Autodesk Inventor part; units mm, degrees
ref_plane "Work Plane1" through (-19.25, -0.5, 9.85) normal (0, 0, 1) x (1, 0, 0)
ref_plane "Work Plane2" through (-19.25, -0.5, 12.85) normal (0, 0, 1) x (1, 0, 0)
ref_plane "Work Plane4" through (19.95, -28.3, 9.85) normal (1, 0, 0) x (0, 0, -1)
ref_plane "Work Plane1" through (-19.25, -0.5, 9.85) normal (0, 0, 1) x (1, 0, 0)
sketch "Sketch1" plane through (-19.25, -0.5, 9.85) normal (0, 0, 1) x (1, 0, 0)
  line L0 (-0.695, -27.8) -> (39.2, -27.8)
  line L1 (39.2, -27.8) -> (39.2, 8.9608)
  line L2 (39.2, 8.9608) -> (-0.695, 8.9608)
  line L3 (-0.695, 8.9608) -> (-0.695, -27.8)
  point P0 (19.25, 0.5)
extrude "Extrusion1" add sketch "Sketch1" along normal blind 3
ref_plane "Work Plane2" through (-19.25, -0.5, 12.85) normal (0, 0, 1) x (1, 0, 0)
sketch "Sketch2" plane through (-19.25, -0.5, 12.85) normal (0, 0, 1) x (1, 0, 0)
  line L0 (39.2, -27.8) -> (39.2, 8.9608)
  line L1 (39.2, -27.8) -> (-0.695, -27.8)
  line L2 (-0.695, -27.8) -> (-0.695, 8.9608)
  line L3 (-0.695, 8.9608) -> (39.2, 8.9608)
  line L4 (39.2, 8.9608) -> (39.2, -27.8)
  point P0 (19.25, 0.5)
  point P1 (39.2, 8.9608)
extrude "Extrusion2" add sketch "Sketch2" along normal blind 5
ref_plane "Work Plane4" through (19.95, -28.3, 9.85) normal (1, 0, 0) x (0, 0, -1)
sketch "Sketch3" plane through (19.95, -28.3, 9.85) normal (1, 0, 0) x (0, 0, -1)
  line L0 (0, 0) -> (0, 36.7608)
  line L1 (0, 0) -> (-8, 0)
  line L2 (0, 36.7608) -> (-2, 36.7608)
  line L3 (-2, 36.7608) -> (-2, 0)
  line L4 (-2, 0) -> (0, 0)
  line L5 (0, 0) -> (0, 36.7608)
  point P0 (9.85, 28.3)
  dimension "d4" = 2
extrude "Extrusion3" cut sketch "Sketch3" against normal blind 50
ref_plane "Work Plane3" through (19.95, -28.3, 17.85) normal (1, 0, 0) x (0, 0, -1)
sketch "Sketch4" plane through (19.95, -28.3, 17.85) normal (1, 0, 0) x (0, 0, -1)
  line L0 (6, 0) -> (0, 0)
  line L1 (6, 36.7608) -> (0, 36.7608)
  line L2 (0, 0) -> (1, 0)
  line L3 (1, 0) -> (1, 36.7608)
  line L4 (1, 36.7608) -> (0, 36.7608)
  line L5 (0, 36.7608) -> (0, 0)
  point P0 (17.85, 28.3)
  point P1 (1, 0)
  dimension "d7" = 1
extrude "Extrusion4" cut sketch "Sketch4" against normal blind 50
ref_plane "Work Plane5" through (19.95, -28.3, 11.85) normal (1, 0, 0) x (0, 0, -1)
sketch "Sketch5" plane through (19.95, -28.3, 11.85) normal (1, 0, 0) x (0, 0, -1)
  line L0 (-5, 36.7608) -> (-5, 0)
  line L1 (0, 0) -> (0, 36.7608)
  line L2 (-5, 36.7608) -> (0, 36.7608)
  line L3 (0, 36.7608) -> (0, 0)
  line L4 (0, 0) -> (-5, 0)
  line L5 (-5, 0) -> (-5, 36.7608)
  point P0 (11.85, 28.3)
extrude "Extrusion5" add sketch "Sketch5" along normal blind 7
ref_plane "Work Plane6" through (-19.945, -28.3, 11.85) normal (0, 0, -1) x (-1, 0, 0)
sketch "Sketch6" plane through (-19.945, -28.3, 11.85) normal (0, 0, -1) x (-1, 0, 0)
  line L0 (-46.895, 0) -> (-46.895, 36.7608)
  line L1 (-46.895, 27.8459) -> (-40.895, 27.8459)
  line L2 (-40.895, 27.8459) -> (-40.895, 11.8459)
  line L3 (-40.895, 11.8459) -> (-46.895, 11.8459)
  line L4 (-46.895, 11.8459) -> (-46.895, 27.8459)
  point P0 (-19.945, 28.3)
  dimension "d12" = 6
  dimension "d13" = 16
extrude "Extrusion6" add sketch "Sketch6" along normal blind 22.875
sketch "Sketch7" plane through (20.95, -0.4541, 11.85) normal (0, 1, 0) x (1, 0, 0)
  arc A0 (5.4164, 8.2173) -> (5.4164, 5.6327) centre (3.7611, 6.925) ccw
  circle A1 centre (3.7611, 6.925) radius 2.5
  arc A2 (5.4164, 18.0673) -> (5.4164, 15.4827) centre (3.7611, 16.775) ccw
  circle A3 centre (3.7611, 16.775) radius 2.5
  point P0 (-20.95, 11.85)
  dimension "d16" = 5
  dimension "d17" = 5
extrude "Extrusion7" cut sketch "Sketch7" against normal blind 22.875
ref_plane "Work Plane7" through (26.95, -28.3, 11.85) normal (1, 0, 0) x (0, 0, -1)
sketch "Sketch8" plane through (26.95, -28.3, 11.85) normal (1, 0, 0) x (0, 0, -1)
  line L0 (0, 11.8459) -> (22.875, 11.8459)
  line L1 (22.875, 27.8459) -> (22.875, 11.8459)
  line L2 (0, 11.8459) -> (22.875, 11.8459)
  line L3 (22.875, 11.8459) -> (22.875, 16.8459)
  line L4 (22.875, 16.8459) -> (0, 16.8459)
  line L5 (0, 16.8459) -> (0, 11.8459)
  point P0 (11.85, 28.3)
  dimension "d20" = 5
extrude "Extrusion8" cut sketch "Sketch8" against normal blind 6.7
ref_plane "Work Plane8" through (-19.945, -28.3, 11.85) normal (-1, 0, 0) x (0, 0, 1)
sketch "Sketch9" plane through (-19.945, -28.3, 11.85) normal (-1, 0, 0) x (0, 0, 1)
  line L0 (0, 36.7608) -> (0, 0)
  line L1 (5, 0) -> (0, 0)
  line L2 (0, 36.7608) -> (5, 36.7608)
  line L3 (5, 36.7608) -> (5, 0)
  line L4 (5, 0) -> (0, 0)
  line L5 (0, 0) -> (0, 36.7608)
  point P0 (-11.85, 28.3)
extrude "Extrusion9" add sketch "Sketch9" along normal blind 7
ref_plane "Work Plane10" through (26.95, -0.4541, 11.85) normal (0, 0, -1) x (-1, 0, 0)
sketch "Sketch11" plane through (26.95, -0.4541, 11.85) normal (0, 0, -1) x (-1, 0, 0)
  line L0 (53.895, -27.8459) -> (53.895, 8.9148)
  line L1 (53.895, 0) -> (47.895, 0)
  line L2 (47.895, 0) -> (47.895, -11)
  line L3 (47.895, -11) -> (53.895, -11)
  line L4 (53.895, -11) -> (53.895, 0)
  point P0 (26.95, 0.4541)
  dimension "d25" = 6
extrude "Extrusion10" add sketch "Sketch11" along normal blind 22.875
sketch "Sketch12" plane through (-26.945, -0.4541, 11.85) normal (0, 1, 0) x (1, 0, 0)
  arc A0 (0.5786, 15.4827) -> (0.5786, 18.0673) centre (2.2339, 16.775) ccw
  circle A1 centre (2.2339, 16.775) radius 2.5
  arc A2 (0.5786, 5.6327) -> (0.5786, 8.2173) centre (2.2339, 6.925) ccw
  circle A3 centre (2.2339, 6.925) radius 2.5
  point P0 (26.945, 11.85)
  dimension "d28" = 5
  dimension "d29" = 5
extrude "Extrusion11" cut sketch "Sketch12" against normal blind 22.875
ref_plane "Work Plane11" through (-26.945, -28.3, 11.85) normal (-1, 0, 0) x (0, 0, 1)
sketch "Sketch13" plane through (-26.945, -28.3, 11.85) normal (-1, 0, 0) x (0, 0, 1)
  line L0 (0, 16.8459) -> (0, 27.8459)
  line L1 (5, 36.7608) -> (0, 36.7608)
  line L2 (0, 27.8459) -> (5, 27.8459)
  line L3 (5, 27.8459) -> (5, 36.7608)
  line L4 (5, 36.7608) -> (0, 36.7608)
  line L5 (0, 36.7608) -> (0, 27.8459)
  point P0 (-11.85, 28.3)
extrude "Extrusion12" cut sketch "Sketch13" against normal blind 67.325
ref_plane "Work Plane9" through (26.95, -28.3, 11.85) normal (0, -1, 0) x (1, 0, 0)
sketch "Sketch14" plane through (26.95, -28.3, 11.85) normal (0, -1, 0) x (1, 0, 0)
  line L0 (0, 5) -> (0, 0)
  line L1 (0, 5) -> (-53.895, 5)
  line L2 (0, 0) -> (-53.895, 0)
  line L3 (-53.895, 0) -> (-53.895, 5)
  line L4 (-53.895, 5) -> (0, 5)
  line L5 (0, 5) -> (0, 0)
  point P0 (-26.95, -11.85)
extrude "Extrusion13" add sketch "Sketch14" along normal blind 5
ref_plane "Work Plane12" through (26.95, -11.4541, 11.85) normal (0, 0, -1) x (-1, 0, 0)
sketch "Sketch15" plane through (26.95, -11.4541, 11.85) normal (0, 0, -1) x (-1, 0, 0)
  line L0 (53.895, -21.8459) -> (0, -21.8459)
  line L1 (53.895, 11) -> (53.895, -21.8459)
  line L2 (0, -21.8459) -> (53.895, -21.8459)
  line L3 (53.895, -21.8459) -> (53.895, -17.8459)
  line L4 (53.895, -17.8459) -> (0, -17.8459)
  line L5 (0, -17.8459) -> (0, -21.8459)
  point P0 (26.95, 11.4541)
  dimension "d36" = 4
extrude "Extrusion14" add sketch "Sketch15" along normal blind 22.4625
ref_plane "Work Plane13" through (-26.945, -29.3, 11.85) normal (0, 1, 0) x (1, 0, 0)
sketch "Sketch16" plane through (-26.945, -29.3, 11.85) normal (0, 1, 0) x (1, 0, 0)
  line L0 (53.895, 0) -> (53.895, 22.4625)
  line L1 (0, 0) -> (0, 22.4625)
  line L2 (53.895, 0) -> (0, 0)
  line L3 (0, 0) -> (0, 1)
  line L4 (0, 1) -> (53.895, 1)
  line L5 (53.895, 1) -> (53.895, 0)
  point P0 (26.945, 11.85)
  point P1 (53.895, 1)
  dimension "d39" = 1
extrude "Extrusion15" add sketch "Sketch16" along normal blind 30
ref_plane "Work Plane14" through (26.95, -28.3, 11.85) normal (1, 0, 0) x (0, 0, -1)
sketch "Sketch17" plane through (26.95, -28.3, 11.85) normal (1, 0, 0) x (0, 0, -1)
  line L0 (0, 29) -> (1, 29)
  line L1 (5.8126, 27.8459) -> (1, 27.8459)
  line L2 (0, 29) -> (1, 29)
  line L3 (1, 29) -> (1, 27.8459)
  line L4 (1, 27.8459) -> (0, 27.8459)
  line L5 (0, 27.8459) -> (0, 29)
  point P0 (11.85, 28.3)
extrude "Extrusion16" cut sketch "Sketch17" against normal blind 100
sketch "Sketch19" plane through (26.95, -33.3, 11.85) normal (0, -1, 0) x (1, 0, 0)
  circle A0 centre (-16.85, -11.85) radius 5
  circle A1 centre (-16.85, -11.85) radius 1.5
  point P0 (-26.95, -11.85)
  dimension "d47" = 10
  dimension "d50" = 3
extrude "Extrusion20" cut sketch "Sketch19" against normal blind 10 contours A1
sketch "Sketch20" plane through (26.95, -33.3, 11.85) normal (0, -1, 0) x (1, 0, 0)
  line L0 (-53.895, -22.4625) -> (0, -22.4625)
  line L1 (-53.895, 5) -> (-53.895, -22.4625)
  line L2 (0, -22.4625) -> (-53.895, -22.4625)
  line L3 (-53.895, -22.4625) -> (-53.895, 5)
  line L4 (-53.895, 5) -> (0, 5)
  line L5 (0, 5) -> (0, -22.4625)
  point P0 (-26.95, -11.85)
extrude "Extrusion21" add sketch "Sketch20" along normal blind 2
sketch "Sketch21" plane through (-26.945, -29.3, -10.6125) normal (0, 1, 0) x (1, 0, 0)
  circle A0 centre (37.045, -10.6125) radius 1.5
  circle A1 centre (37.045, -10.6125) radius 1.5
  point P0 (26.945, -10.6125)
extrude "Extrusion22" cut sketch "Sketch21" against normal blind 10
sketch "Sketch22" plane through (-26.945, -29.3, -10.6125) normal (0, 1, 0) x (1, 0, 0)
  circle A0 centre (37.045, -10.6125) radius 1.5
  circle A1 centre (37.045, -10.6125) radius 2.5
  point P0 (26.945, -10.6125)
  dimension "d59" = 5
extrude "Extrusion23" cut sketch "Sketch22" against normal blind 2
sketch "Sketch23" plane through (-19.945, -28.3, -11.025) normal (0, 0, -1) x (-1, 0, 0)
  line L0 (-46.895, 27.8459) -> (-46.895, 16.8459)
  line L1 (-46.895, 27.8459) -> (-48.895, 27.8459)
  line L2 (-48.895, 27.8459) -> (-48.895, 16.8459)
  line L3 (-48.895, 16.8459) -> (-46.895, 16.8459)
  line L4 (-46.895, 16.8459) -> (-46.895, 27.8459)
  line L5 (7, 16.8459) -> (7, 27.8459)
  line L6 (7, 27.8459) -> (9, 27.8459)
  line L7 (9, 27.8459) -> (9, 16.8459)
  line L8 (9, 16.8459) -> (7, 16.8459)
  line L9 (7, 16.8459) -> (7, 27.8459)
  point P0 (-19.945, 28.3)
  dimension "d62" = 2
  dimension "d63" = 2
extrude "Extrusion24" add sketch "Sketch23" against normal up to surface (27.875 mm away)
sketch "Sketch24" plane through (-20.945, -0.4541, 10.85) normal (0, 1, 0) x (1, 0, 0)
  arc A0 (47.895, 7.0374) -> (47.895, 4.8126) centre (45.6561, 5.925) ccw
  circle A1 centre (45.6561, 5.925) radius 1.6
  arc A2 (47.895, 16.8874) -> (47.895, 14.6626) centre (45.6561, 15.775) ccw
  circle A3 centre (45.6561, 15.775) radius 1.6
  circle A4 centre (45.6561, 5.925) radius 2.5
  circle A5 centre (45.6561, 15.775) radius 2.5
  point P0 (20.945, 10.85)
  point P1 (47.895, 4.8126)
  dimension "d66" = 3.2
  dimension "d67" = 3.2
extrude "Extrusion25" add sketch "Sketch24" against normal up to surface (11 mm away)
sketch "Sketch25" plane through (-20.945, -0.4541, 10.85) normal (0, 1, 0) x (1, 0, 0)
  arc A0 (-6, 4.8025) -> (-6, 7.0475) centre (-3.7661, 5.925) ccw
  circle A1 centre (-3.7661, 5.925) radius 1.6
  arc A2 (-6, 14.6525) -> (-6, 16.8975) centre (-3.7661, 15.775) ccw
  circle A3 centre (-3.7661, 15.775) radius 1.6
  circle A4 centre (-3.7661, 15.775) radius 2.5
  circle A5 centre (-3.7661, 5.925) radius 2.5
  point P0 (20.945, 10.85)
  point P1 (-6, 7.0475)
  dimension "d70" = 3.2
  dimension "d71" = 3.2
  dimension "d72" = 5
  dimension "d73" = 5
extrude "Extrusion26" add sketch "Sketch25" against normal up to surface (11 mm away)
sketch "Sketch26" plane through (26.95, -35.3, 11.85) normal (0, -1, 0) x (1, 0, 0)
  line L0 (-55.895, -22.875) -> (-55.895, 5)
  line L1 (-55.895, -11.85) -> (-37.045, -11.85)
  line L2 (-55.895, -11.85) -> (-37.045, -11.85) construction
  circle A0 centre (-37.045, -11.85) radius 1.5
  point P0 (-26.95, -11.85)
  dimension "d76" = 18.85
  dimension "d77" = 0
  dimension "d78" = 3
extrude "Extrusion27" cut sketch "Sketch26" against normal blind 10
sketch "Sketch27" plane through (-26.945, -29.3, -10.6125) normal (0, 1, 0) x (1, 0, 0)
  circle A0 centre (16.85, -10.6125) radius 1.5
  circle A1 centre (16.85, -10.6125) radius 2.5
  point P0 (26.945, -10.6125)
  dimension "d81" = 5
extrude "Extrusion28" cut sketch "Sketch27" against normal up to surface (2 mm away)
sketch "Sketch28" plane through (-26.945, -35.3, 16.85) normal (0, 0, 1) x (1, 0, 0)
  line L0 (0, 0) -> (53.895, 0)
  line L1 (26.9475, 0) -> (26.9475, 34.8459)
  line L2 (6, 34.8459) -> (47.895, 34.8459)
  point P0 (26.945, 35.3)
sketch "Sketch29" plane through (-26.945, -11.4541, 10.85) normal (0, -1, 0) x (1, 0, 0)
  line L0 (6, 0) -> (0, 0)
  line L1 (-2, 6) -> (0, 6)
  line L2 (0, 0) -> (-2, 0)
  line L3 (-2, 0) -> (-2, 6)
  line L4 (-2, 6) -> (0, 6)
  line L5 (0, 6) -> (0, 0)
  line L6 (53.895, 0) -> (53.895, 6)
  line L7 (55.895, -21.875) -> (55.895, 6)
  line L8 (53.895, 0) -> (55.895, 0)
  line L9 (55.895, 0) -> (55.895, 6)
  line L10 (55.895, 6) -> (53.895, 6)
  line L11 (53.895, 6) -> (53.895, 0)
  point P0 (26.945, -10.85)
extrude "Extrusion29" add sketch "Sketch29" along normal up to surface (23.8459 mm away)
sketch "Sketch30" plane through (26.95, -29.3, 10.85) normal (0, 0, -1) x (-1, 0, 0)
  line L0 (53.895, 0) -> (0, 0)
  line L1 (-2, -6) -> (0, -6)
  line L2 (0, 0) -> (-2, 0)
  line L3 (-2, 0) -> (-2, -6)
  line L4 (-2, -6) -> (0, -6)
  line L5 (0, -6) -> (0, 0)
  line L6 (55.895, -6) -> (-2, -6)
  line L7 (55.895, 17.8459) -> (55.895, -6)
  line L8 (53.895, -6) -> (55.895, -6)
  line L9 (55.895, -6) -> (55.895, 0)
  line L10 (55.895, 0) -> (53.895, 0)
  line L11 (53.895, 0) -> (53.895, -6)
  point P0 (26.95, 29.3)
extrude "Extrusion30" add sketch "Sketch30" along normal up to surface (21.4625 mm away) contours L10 L7 L6 L11 | L5 L1 L3 L2
properties part number "MG996RServoHolder" material "钢"
For this review, take the finished solid that the model builds, in its own axes (mm). A direction names the side the tool comes from. Give positions to 0.01 mm unless a question says otherwise; leave off trailing zeros. Loops run counter-clockwise (first coordinate to the right, second up) from the corner with the lowest first, then second, coordinate; pieces in that order, holes last. Notation, with made-up numbers: M 7.5,57.5 L 61.5,57.5 A26 ccw 61.5,78.5 Z; hole C 36,-29 d4. An arc over 180 degrees is marked long. Answer as a JSON object with one key per item and string values. Group by question number.
Q1. Mouldability with a two-part tool opening along Z and no side actions: class faces 1 (the cylindrical face through (23.532, -5.877, 3.844)), 2 (the flat face through (28.95, -10, 6)), 3 (the flat face through (0, -15, 10.85)) as +Z half, -Z half, draft (parallel to the pull), parting line (faces both ways), or undercut.
Q2. Add section B-B on x = 10.1. Give the boundary of the cut face in (y, z).
Q3. Add section C-C on y = -5.5. Give the boundary of the cut face in (x, z) (3 decimals).
Q4. Add section D-D on x = 20. Give the boundary of the cut face in (y, z), and give its area (3 significant figures).
Q5. Tool access review of faces 4 (the flat face through (0, -0.454, 12)), 5 (the flat face through (0, -29.3, 0)), 6 (the cylindrical face through (-23.973, -5.877, -3.506)), 7 (the flat face through (0, -32, -10.612)): name each direction out of +Z, -Z, +X, -X, +Y, -Y from which nothing blocks a thin tool from reaching the whole face with its end or side.
Q6. Insertion check: P1, Ø2.5, axis at x = -24.71, z = 4.92, coming from the +Y side; P2, Ø1.8, axis at x = 10.1, z = 0, coming from the +Y side; P3, Ø14.5, axis at x = 0, y = -8, coming from the -Z side; P4, Ø1.5, axis at x = -9.5, z = 1, coming from the +Y side. Each pin has a flat end and moves straight along its axis. Give the tip position at first contact, or say it passes through.
Q7. For probe 1 along X at (y, z) = (-34.2, 0) (3 decimals); probe 2 along Y at (x, z) = (26, 0.75); probe 3 along X at (y, z) = (-4, 2.75) (3 decimals), list the stretches that pass through material, from the lowest coordinate up. Write a range as [from, to].
Q8. Add section A-A on z = 0. Give the boundary of the cut face in (x, y) (3 decimals), and give its area (3 significant figures).
Checked values:
{
 "1": {"face 1": "undercut", "face 2": "draft", "face 3": "-Z half"},
 "2": {"outline": "M -35.3,-10.61 L -29.3,-10.61 L -29.3,-2.5 L -31.3,-2.5 L -31.3,-1.5 L -35.3,-1.5 Z; M -35.3,1.5 L -31.3,1.5 L -31.3,2.5 L -29.3,2.5 L -29.3,10.85 L -0.45,10.85 L -0.45,16.85 L -35.3,16.85 Z"},
 "3": {"outline": "M -28.945,-11.025 L -20.945,-11.025 L -20.945,10.85 L 20.95,10.85 L 20.95,-11.025 L 28.95,-11.025 L 28.95,16.85 L -28.945,16.85 Z; hole C -24.711,-4.925 d3.2; hole C -24.711,4.925 d3.2; hole C 24.711,-4.925 d3.2; hole C 24.711,4.925 d3.2"},
 "4": {"outline": "M -35.3,-10.61 L -29.3,-10.61 L -29.3,10.85 L -0.45,10.85 L -0.45,16.85 L -35.3,16.85 Z", "area": "338 mm²"},
 "5": {"face 4": "+Z, -Z, +X, -X, +Y", "face 5": "-Z, +X, -X", "face 6": "+Y", "face 7": "-Z, +X, -X, -Y"},
 "6": {"P1": "y = -29.3", "P2": "through", "P3": "z = 10.85", "P4": "y = -31.3"},
 "7": {"probe 1": "[-28.945, -11.595], [-8.595, 8.6], [11.6, 28.95]", "probe 2": "[-35.3, -29.3], [-11.45, -0.45]", "probe 3": "[-28.945, -20.945], [20.95, 28.95]"},
 "8": {"outline": "M -28.945,-35.3 L -11.595,-35.3 L -11.595,-31.3 L -12.595,-31.3 L -12.595,-29.3 L -28.945,-29.3 Z; M -28.945,-11.454 L -20.945,-11.454 L -20.945,-0.454 L -28.945,-0.454 Z; M -8.595,-35.3 L 8.6,-35.3 L 8.6,-31.3 L 7.6,-31.3 L 7.6,-29.3 L -7.595,-29.3 L -7.595,-31.3 L -8.595,-31.3 Z; M 11.6,-35.3 L 28.95,-35.3 L 28.95,-29.3 L 12.6,-29.3 L 12.6,-31.3 L 11.6,-31.3 Z; M 20.95,-11.454 L 28.95,-11.454 L 28.95,-0.454 L 20.95,-0.454 Z", "area": "479 mm²"}
}
